Answer from the drawing. Dimensions are ordinates in mm from the lowest x, y and z of the part. A direction names the side the tool comes from. Give positions to 0.01 mm unless a question says otherwise; leave off trailing zeros. Loops run counter-clockwise (first coordinate to the right, second up) from the corner with the lowest first, then second, coordinate; pieces in that order, holes last. Notation, with made-up numbers: (13, 8.5) - (37, 8.5) arc R5 ccw to (37, 17.5) - close; hole circle Ø4 at (61.5, 50). An arc over 180 degrees is marked (long way). Answer as CSV lines item,"result". Start each with the question number.
1) Find the intervals of material crossed by line 1 along Z through (x, y) = (7, 13.05); line 2 along Y through (x, z) = (7, 9); line 3 along Z through (x, y) = (7, 11.4), in increasing order.
2) Flat-ended cylindrical pins translate along their axes: pin 1 (2 mm diameter, centred on y = 5.5, z = 13, fed in from +X); pin 2 (4 mm diameter, centred on x = 10.5, z = 13.5, fed in from -Y); pin 3 (3 mm diameter, centred on y = 4.5, z = 22, fed in from -X). Find the tip coordinate at first contact, or state that the pin passes through.
3) A cutting plane is placed at B-B (z = 8.25). Determine the outline of the cut face in (x, y), and give its area (3 significant figures).
4) For the marked faces 1 and 2, determine the directions among +Z, -Z, +X, -X, +Y, -Y from which every point of the face is accessible in a straight line to the end or side of a thin tool.
5) A cutting plane is placed at A-A (x = 7). Give the number of separate pieces and of enclosed holes in the cut face, and give its area (3 significant figures).
6) For a pull along X with two mould halves and no side action, classify the marked faces 3 and 4 as pulls with the +X half, pulls with the -X half, needs draft (parallel to the pull), parting line crosses it, or undercut.
7) A cutting plane is placed at C-C (z = 20.4). Determine the outline of the cut face in (x, y).
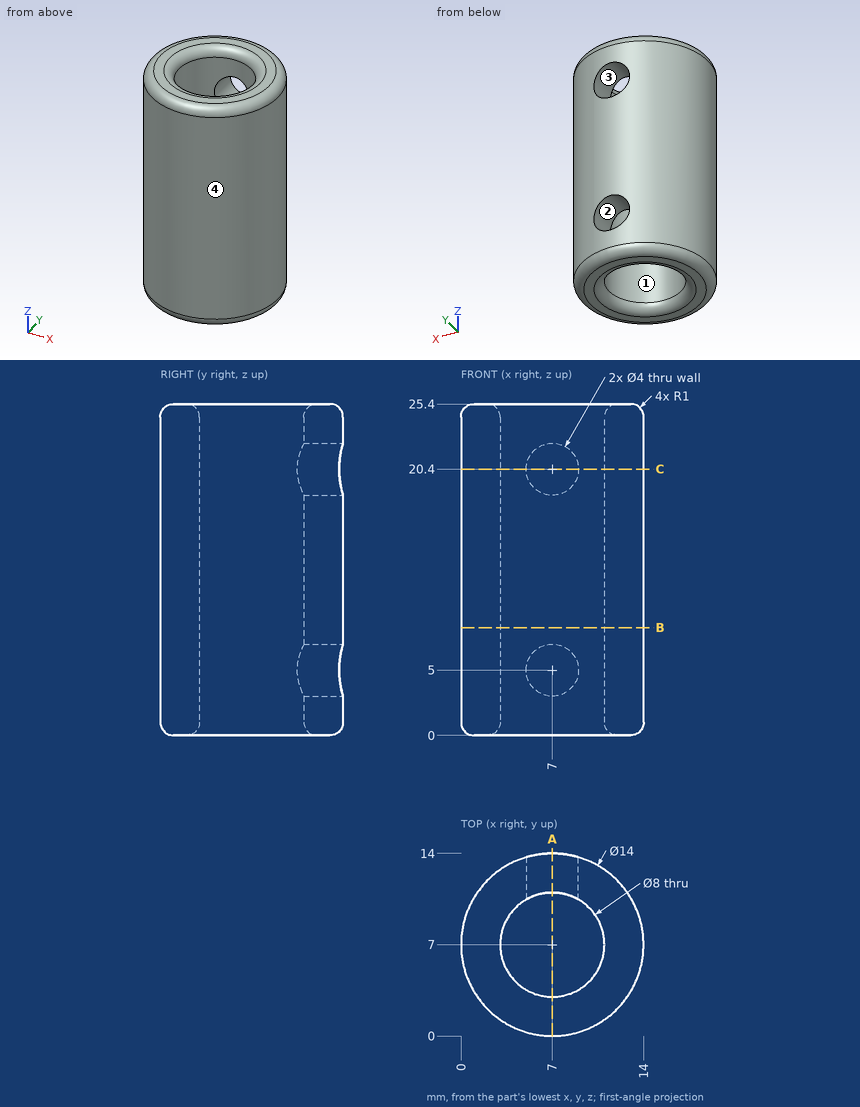
Ans:
1,line 1,"0 to 3, 7 to 18.4, 22.4 to 25.4"
1,line 2,"0 to 3, 11 to 14"
1,line 3,"0.2 to 3, 7 to 18.4, 22.4 to 25.2"
2,pin 1,"x = 13.98"
2,pin 2,"y = 0.16"
2,pin 3,"x = 0.07"
3,outline,"circle Ø14 at (7, 7); hole circle Ø8 at (7, 7)"
3,area,"104 mm2"
4,face 1,"+Z, -Z"
4,face 2,"+Y"
5,separate pieces,"4"
5,enclosed holes,"0"
5,area,"127 mm2"
6,face 3,"undercut"
6,face 4,"parting line crosses it"
7,outline,"(5, 10.46) - (5, 13.71) arc R7 ccw (long way) to (9, 13.71) - (9, 10.46) arc R4 cw (long way) to start"
